Input: part model. Units: mm. Frame: model coordinates. A direction names the side the tool comes from. Round coordinates to 2 decimals unless told otherwise and drop trailing zeros. Order: outer loops, then holes, each group sorted by start corner. A loop starts at its lowest first (then second) coordinate and runs counter-clockwise, first axis right, second up. Notation, with made-up numbers: (41, 43) -> (96, 43) arc R24 ccw to (96, 59) -> close; hole circle Ø3 at (80.25, 68). An arc over 180 degrees is marked (long way). Use a Markdown table: item, result.
from build123d import *

# Parameters (mm, degrees)
EXTRUDE_1_DEPTH        = 12
SKETCH_2_W             = 1706
SKETCH_2_H             = 12
EXTRUDE_2_DEPTH        = 190
EXTRUDE_3_DEPTH        = 12
SKETCH_4_W             = 430
SKETCH_4_H             = 12
EXTRUDE_4_DEPTH        = 502
SKETCH_5_R             = 30
SKETCH_5_R_2           = 6
CUT_EXTRUDE_1_DEPTH    = 1065.139088653
SKETCH_6_W             = 10
SKETCH_6_H             = 165
EXTRUDE_5_DEPTH        = 38
CUT_EXTRUDE_2_DEPTH    = 10
SKETCH_8_W             = 10
SKETCH_8_H             = 210
EXTRUDE_6_DEPTH        = 190
SKETCH_9_W             = 10
SKETCH_9_H             = 38
EXTRUDE_7_DEPTH        = 220
CUT_EXTRUDE_3_DEPTH    = 18
PATTERN_LINEAR_1_COUNT = 2
PATTERN_LINEAR_1_PITCH = 270
SKETCH_11_W            = 12
SKETCH_11_H            = 234
SKETCH_11_H_2          = 210
EXTRUDE_8_DEPTH        = 190
SKETCH_12_R            = 75
SKETCH_12_R_2          = 30
SKETCH_12_R_3          = 6
EXTRUDE_9_DEPTH        = 10
PATTERN_LINEAR_2_COUNT = 2
PATTERN_LINEAR_2_PITCH = 200
SKETCH_14_W            = 10
SKETCH_14_H            = 210
EXTRUDE_10_DEPTH       = 100


with BuildPart() as part:
    # 草图1 → 凸台-拉伸1 (new body)
    with BuildSketch(Plane(origin=(0, 0, 0), x_dir=(1, 0, 0), z_dir=(0, 1, 0))):
        with BuildLine():
            Line((-898, 155), (898, 155))
            Line((898, 155), (898, 75))
            Line((898, 75), (878, 75))
            ThreePointArc((878, 75), (803, 0), (878, -75))
            Line((878, -75), (898, -75))
            Line((898, -75), (898, -155))
            Line((898, -155), (-898, -155))
            Line((-898, -155), (-898, -75))
            Line((-898, -75), (-878, -75))
            ThreePointArc((-878, -75), (-803, 0), (-878, 75))
            Line((-878, 75), (-898, 75))
            Line((-898, 75), (-898, 155))
        make_face()
    extrude(amount=EXTRUDE_1_DEPTH)

    # 草图2 → 凸台-拉伸2 (add)
    with BuildSketch(Plane(origin=(0, 0, 0), x_dir=(-1, 0, 0), z_dir=(0, -1, 0))):
        with Locations((0, 134)):
            Rectangle(SKETCH_2_W, SKETCH_2_H)
        with Locations((0, -134)):
            Rectangle(SKETCH_2_W, SKETCH_2_H)
    extrude(amount=EXTRUDE_2_DEPTH)

    # 草图3 → 凸台-拉伸3 (add)
    with BuildSketch(Plane.XZ.offset(190)):
        with BuildLine():
            Line((-878, 155), (878, 155))
            Line((878, 155), (878, 15))
            ThreePointArc((878, 15), (863, 0), (878, -15))
            Line((878, -15), (878, -155))
            Line((878, -155), (-878, -155))
            Line((-878, -155), (-878, -15))
            ThreePointArc((-878, -15), (-863, 0), (-878, 15))
            Line((-878, 15), (-878, 155))
        make_face()
    extrude(amount=EXTRUDE_3_DEPTH)

    # 草图4 → 凸台-拉伸4 (add)
    with BuildSketch(Plane(origin=(0, 0, 0), x_dir=(-1, 0, 0), z_dir=(0, -1, 0))):
        with Locations((0, -111)):
            Rectangle(SKETCH_4_W, SKETCH_4_H)
        with Locations((0, 111)):
            Rectangle(SKETCH_4_W, SKETCH_4_H)
    extrude(amount=EXTRUDE_4_DEPTH)

    # 草图5 → 切除-拉伸1 (cut, through all)
    with BuildSketch(Plane(origin=(0, 0, -117), x_dir=(-1, 0, 0), z_dir=(0, 0, -1))):
        with Locations((0, -405)):
            Circle(SKETCH_5_R)
        with Locations((-45, -440)):
            Circle(SKETCH_5_R_2)
        with Locations((45, -440)):
            Circle(SKETCH_5_R_2)
        with BuildLine():
            Line((-215, -382), (-215, -502))
            Line((-215, -502), (215, -502))
            Line((215, -502), (215, -382))
            Line((215, -382), (34.918275337, -473.627356408))
            ThreePointArc((34.918275337, -473.627356408), (0, -482), (-34.918275337, -473.627356408))
            Line((-34.918275337, -473.627356408), (-215, -382))
        make_face()
    extrude(amount=-CUT_EXTRUDE_1_DEPTH, mode=Mode.SUBTRACT)

    # 草图6 → 凸台-拉伸5 (add)
    with BuildSketch(Plane.XY.offset(117)):
        with Locations((0, -284.5)):
            Rectangle(SKETCH_6_W, SKETCH_6_H)
    extrude_5 = extrude(amount=EXTRUDE_5_DEPTH)

    # 镜向1: 凸台-拉伸5 across plane
    add(extrude_5.mirror(Plane.XY))

    # 草图7 → 切除-拉伸2 (cut)
    with BuildSketch(Plane.ZY.offset(5)):
        Polygon((-155, -202), (-155, -367), (-141, -367), align=None)
        Polygon((155, -202), (141, -367), (155, -367), align=None)
    extrude(amount=-CUT_EXTRUDE_2_DEPTH, mode=Mode.SUBTRACT)

    # 草图8 → 凸台-拉伸6 (add)
    with BuildSketch(Plane(origin=(0, -202, 0), x_dir=(-1, 0, 0), z_dir=(0, -1, 0))):
        with Locations((135, 0)):
            Rectangle(SKETCH_8_W, SKETCH_8_H)
        with Locations((-135, 0)):
            Rectangle(SKETCH_8_W, SKETCH_8_H)
    extrude(amount=EXTRUDE_6_DEPTH)

    # 草图9 → 凸台-拉伸7 (add)
    with BuildSketch(Plane(origin=(0, -202, 0), x_dir=(-1, 0, 0), z_dir=(0, -1, 0))):
        with Locations((135, -136)):
            Rectangle(SKETCH_9_W, SKETCH_9_H)
        with Locations((-135, -136)):
            Rectangle(SKETCH_9_W, SKETCH_9_H)
        with Locations((135, 136)):
            Rectangle(SKETCH_9_W, SKETCH_9_H)
        with Locations((-135, 136)):
            Rectangle(SKETCH_9_W, SKETCH_9_H)
    extrude(amount=EXTRUDE_7_DEPTH)

    # 草图10 → 切除-拉伸3 (cut)
    with BuildSketch(Plane(origin=(140, 0, 0), x_dir=(0, 0, -1), z_dir=(1, 0, 0))):
        Polygon((-155, -202), (-155, -422), (-137, -422), align=None)
        Polygon((155, -202), (155, -422), (137, -422), align=None)
    cut_extrude_3 = extrude(amount=-CUT_EXTRUDE_3_DEPTH, mode=Mode.SUBTRACT)

    # 阵列(线性)1: 切除-拉伸3 ×2
    with Locations(*[(-i * PATTERN_LINEAR_1_PITCH, 0, 0) for i in range(1, PATTERN_LINEAR_1_COUNT)]):
        add(cut_extrude_3, mode=Mode.SUBTRACT)

    # 草图11 → 凸台-拉伸8 (add)
    with BuildSketch(Plane(origin=(0, 0, 0), x_dir=(-1, 0, 0), z_dir=(0, -1, 0))):
        with Locations((-221, 0)):
            Rectangle(SKETCH_11_W, SKETCH_11_H)
        with Locations((221, 0)):
            Rectangle(SKETCH_11_W, SKETCH_11_H)
        with Locations((136, 0)):
            Rectangle(SKETCH_11_W, SKETCH_11_H_2)
        with Locations((-136, 0)):
            Rectangle(SKETCH_11_W, SKETCH_11_H_2)
    extrude(amount=EXTRUDE_8_DEPTH)

    # 草图12 → 凸台-拉伸9 (add)
    with BuildSketch(Plane.XY.offset(-105)):
        with Locations(Location((0, -405, 0), (0, 0, 180))):
            Circle(SKETCH_12_R)
        with Locations(Location((0, -405, 0), (0, 0, 180))):
            Circle(SKETCH_12_R_2, mode=Mode.SUBTRACT)
        with Locations(Location((-45, -440, 0), (0, 0, 180))):
            Circle(SKETCH_12_R_3, mode=Mode.SUBTRACT)
        with Locations(Location((45, -440, 0), (0, 0, 180))):
            Circle(SKETCH_12_R_3, mode=Mode.SUBTRACT)
    extrude_9 = extrude(amount=EXTRUDE_9_DEPTH)

    # 阵列(线性)2: 凸台-拉伸9 ×2
    with Locations(*[(0, 0, i * PATTERN_LINEAR_2_PITCH) for i in range(1, PATTERN_LINEAR_2_COUNT)]):
        add(extrude_9)

    # 草图14 → 凸台-拉伸10 (add)
    with BuildSketch(Plane(origin=(0, -202, 0), x_dir=(-1, 0, 0), z_dir=(0, -1, 0))):
        with Locations((65, 0)):
            Rectangle(SKETCH_14_W, SKETCH_14_H)
        with Locations((-65, 0)):
            Rectangle(SKETCH_14_W, SKETCH_14_H)
    extrude(amount=EXTRUDE_10_DEPTH)


solid = part.part
1) Draft query along Z for faces 1 (the face through (178, -310, -117)), 2 (the face through (60, -251, 1)), 3 (the face through (-5, -286, -132)). Return one class per face: released by +Z, released by -Z, zero draft, split by the parting line, or undercut.
Answer key:
| item | result |
|---|---|
| face 1 | released by -Z |
| face 2 | undercut |
| face 3 | zero draft |
2) Cut plane B-B on x = -609. Return loops of the section in (y, z), and give its area (3 significant figures).
Answer key:
| item | result |
|---|---|
| outline | (-202, -155) -> (-190, -155) -> (-190, -140) -> (0, -140) -> (0, -155) -> (12, -155) -> (12, 155) -> (0, 155) -> (0, 140) -> (-190, 140) -> (-190, 155) -> (-202, 155) -> close; hole (-190, -128) -> (0, -128) -> (0, 128) -> (-190, 128) -> close |
| area | 12,000 mm^2 |
3) Cut plane A-A on y = -135.5. Return loops of the section in (x, z), and give its area (3 significant figures).
Answer key:
| item | result |
|---|---|
| outline | (-853, -140) -> (853, -140) -> (853, -128) -> (-853, -128) -> close; (-853, 128) -> (853, 128) -> (853, 140) -> (-853, 140) -> close; (-227, -117) -> (227, -117) -> (227, 117) -> (-227, 117) -> close; hole (-215, -105) -> (-142, -105) -> (-142, 105) -> (-215, 105) -> close; hole (-130, -105) -> (130, -105) -> (130, 105) -> (-130, 105) -> close; hole (142, -105) -> (215, -105) -> (215, 105) -> (142, 105) -> close |
| area | 61,900 mm^2 |
4) Contact query for flat-ended pins moving along their axis: P1, Ø13, axis at y = -198, z = -91.5, coming from the -X side; P2, Ø8, axis at y = -178, z = 99.5, coming from the -X side; P3, Ø8, axis at x = 133.5, z = 56.5, coming from the -Y side. Output: stop coordinate, or through.
Answer key:
| item | result |
|---|---|
| P1 | stops at x = -878 |
| P2 | stops at x = -227 |
| P3 | stops at y = -392 |
5) Ray query, probe 1 along X at (y, z) = (-224, 84.5); probe 2 along Y at (x, z) = (-646, 109.5); probe 3 along Z at (x, y) = (78, -424.5). Return the intervals inside material, ascending.
Answer key:
| item | result |
|---|---|
| probe 1 | x = -140 to -130, -70 to -60, 60 to 70, 130 to 140 |
| probe 2 | y = -202 to -190, 0 to 12 |
| probe 3 | z = -117 to -105, 105 to 117 |
6) Set-up query: faces 4 (the face through (-130, -310, 132)), 5 (the face through (3, -94, -117)), 6 (the face through (130, -296, 1)). Return all of +Z, -Z, +X, -X, +Y, -Y with unobstructed straight access to the full face (end or side cutting, diameter ignored); none if empty.
Answer key:
| item | result |
|---|---|
| face 4 | +Z, -Y |
| face 5 | +X, -X |
| face 6 | -Y |
7) Cut plane C-C on y = -278. State how many separate pieces and enclosed holes the cut face has, and give its area (3 significant figures).
Answer key:
| item | result |
|---|---|
| separate pieces | 1 |
| enclosed holes | 3 |
| area | 20,600 mm^2 |
